Input: part model. Units: mm. Frame: model coordinates. A direction names the side the tool comes from. Coordinates: 2 decimals unless noted, no trailing zeros. Write each loop counter-clockwise with the first axis right and the second up, starting at its lowest first coordinate (ties: lowest second). Pieces come first, ordered by that corner, then holes. Notation, with made-up numbers: (16.5, -7) -> (37.5, -7) arc R26 ccw to (37.5, 25) -> close; hole circle Ø4 at (45, 27). An arc over 180 degrees is marked (long way). Use one line per item in the form item = value. Start each with the question number.
(1) Set-up query: faces 1 (the face through (0, 0, -38.1)), 2 (the face through (3, 3, 0)). Return all of +Z, -Z, +X, -X, +Y, -Y with unobstructed straight access to the full face (end or side cutting, diameter ignored); none if empty.
(2) Cut plane B-B on y = 1.25. Return the cut outline in (x, z) (3 decimals), plus the area to 3 significant figures.
(3) First-contact query: pin 1 (3 mm diameter, centred on y = -2, z = -10.5, fed in from +X); pin 2 (6 mm diameter, centred on y = -0.5, z = -27.5, fed in from -X) (3 decimals); pin 3 (5 mm diameter, centred on y = 4, z = -8.5, fed in from -X); pin 4 (1.5 mm diameter, centred on x = -5, z = -21.5, fed in from +Y). Flat tips, straight axial feed; report the tip coordinate or a pass-through.
(4) Ray query, line 1 along Z through (x, y) = (-2.75, 4.25) (3 decimals); line 2 along X through (y, z) = (-1.75, -27.5); line 3 along X through (y, z) = (-1.5, -17.5). Return the intervals inside material, ascending.
(5) Cut plane C-C on z = -4.5. Return the cut outline in (x, y) (3 decimals).
(6) Cut plane A-A on x = 0. Return the cut outline in (y, z) (1 decimal), plus the area to 3 significant figures.
(7) Cut plane D-D on x = -4. Return the cut outline in (y, z) (3 decimals).
Autodesk Inventor part; units mm, degrees
ref_plane "YZ Plane" through (0, 0, 0) normal (1, 0, 0) x (0, 1, 0)
ref_plane "XZ Plane" through (0, 0, 0) normal (0, 1, 0) x (-1, 0, 0)
ref_plane "XY Plane" through (0, 0, 0) normal (0, 0, 1) x (1, 0, 0)
sketch "Sketch1" plane through (0, 0, 0) normal (0, 0, 1) x (1, 0, 0)
  circle A0 centre (0, 0) radius 3.175
  line L0 (3.2079, 5.5563) -> (6.4158, 0)
  line L1 (6.4158, 0) -> (3.2079, -5.5562)
  line L2 (3.2079, -5.5562) -> (-3.2079, -5.5562)
  line L3 (-3.2079, -5.5562) -> (-6.4158, 0)
  line L4 (-6.4158, 0) -> (-3.2079, 5.5563)
  line L5 (-3.2079, 5.5563) -> (3.2079, 5.5563)
  dimension "d0" = 6.35
  dimension "d1" = 11.1125
extrude "Extrusion1" add sketch "Sketch1" against normal blind 38.1 contours A0
extrude "Extrusion2" add sketch "Sketch1" along normal blind 3.175 contours A0 | L0 L1 L2 L3 L4 L5
thread "Thread1"
chamfer "Chamfer1" distance 0.7937 angle 45 6 edges at (4.8119, 2.7781, 3.175) (0, 5.5563, 3.175) (-4.8119, 2.7781, 3.175) (-4.8119, -2.7781, 3.175) (0, -5.5562, 3.175) (4.8119, -2.7781, 3.175)
properties part number "1.5_bolt_.25_20"
Values:
q1.face_1 = -Z, +X, -X, +Y, -Y
q1.face_2 = -Z
q2.outline = (-5.694, 0) -> (-2.919, 0) -> (-2.919, -38.1) -> (2.919, -38.1) -> (2.919, 0) -> (5.694, 0) -> (5.694, 2.381) -> (4.778, 3.175) -> (-4.778, 3.175) -> (-5.694, 2.381) -> close
q2.area = 258 mm2
q3.pin_1 = 3.14
q3.pin_2 = -3.175
q3.pin_3 = -2.8
q3.pin_4 = through
q4.line_1 = 0 to 3.175
q4.line_2 = -2.65 to 2.65
q4.line_3 = -2.8 to 2.8
q5.outline = circle Ø6.35 at (0, 0)
q6.outline = (-5.6, 0) -> (-3.2, 0) -> (-3.2, -38.1) -> (3.2, -38.1) -> (3.2, 0) -> (5.6, 0) -> (5.6, 2.4) -> (4.8, 3.2) -> (-4.8, 3.2) -> (-5.6, 2.4) -> close
q6.area = 277 mm2
q7.outline = (-4.184, 0) -> (4.184, 0) -> (4.184, 2.381) -> (2.597, 3.175) -> (-2.597, 3.175) -> (-4.184, 2.381) -> close
